Answer from the drawing. Dimensions are ordinates in mm from the lowest x, y and z of the part. Round coordinates to 2 decimals unless told otherwise and drop trailing zeros. Write each loop counter-clockwise with the first axis right and the second up, starting at its lowest first coordinate (ties: lowest second). Pieces come first, ordered by that corner, then holes. Notation, with made-up numbers: (43, 37.5) -> (63, 37.5) arc R13 cw to (63, 51.5) -> close; hole circle Ø4 at (-38, 20.25). An arc over 180 degrees is marked (long way). Return JSON: item names as keys, results as strings. Group by question number.
(1) Straight lines are drawn through the part: line 1 (Y direction, x = 21, z = 4.75); line 2 (Y direction, x = 15.75, z = 1.25); line 3 (Z direction, x = 23.25, y = 8). For each, find the intervals that lie inside material, in ascending order.
(2) A cutting plane is placed at A-A on x = 12.7. Give the vertices of the cut face in (y, z), then the cut area to 3 significant figures.
(3) The mould has two halves that part along X. Classify the marked faces 1, 2, 3 and 4: released by +X, released by -X, zero draft, split by the parting line, or undercut.
(4) Given pin 1 (6 mm diameter, centred on y = 19.5, z = 12.5, fed in from +X), flat-ended and moving along its own axis, determine where the tip first touches the part or whether it passes through.
(5) A cutting plane is placed at C-C on z = 21.75. Give the vertices of the cut face in (x, y).
(6) A cutting plane is placed at D-D on y = 3.5. Give the vertices of the cut face in (x, z), then the cut area to 3 significant figures.
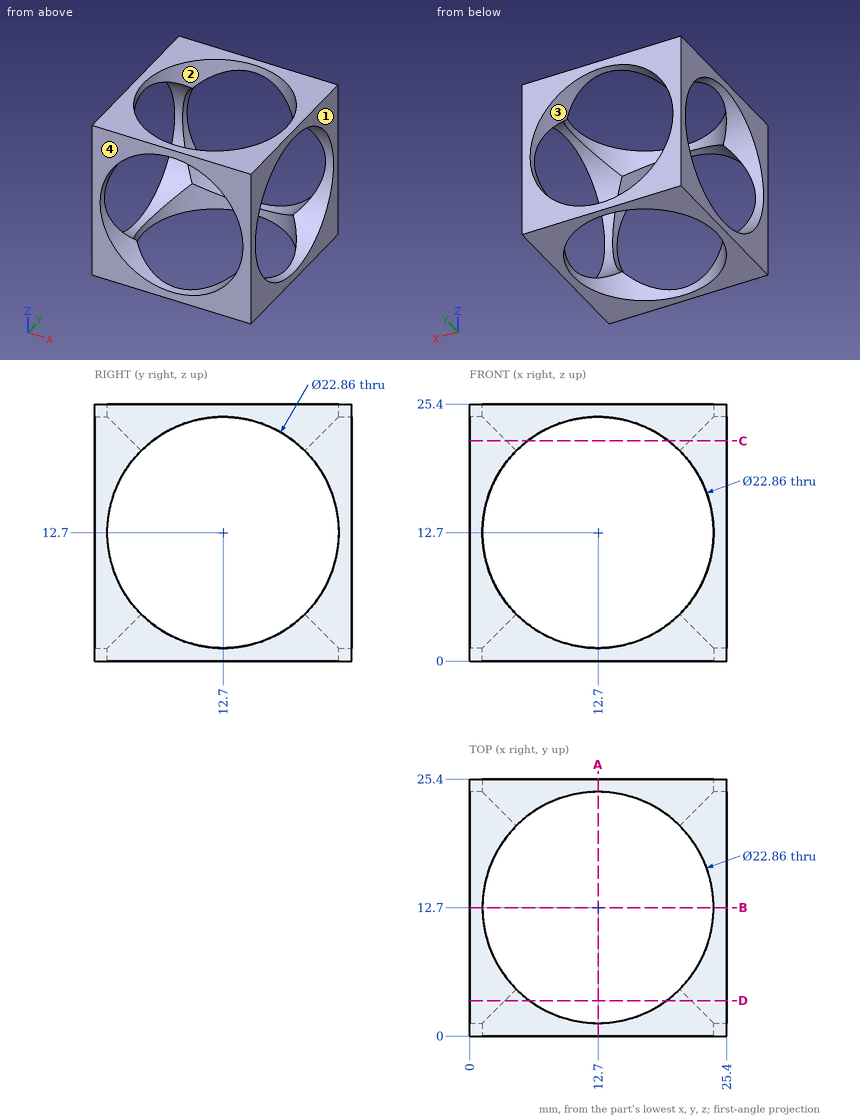
Checks:
{
 "1": {"line 1": "y = 0 to 4.49, 20.91 to 25.4", "line 2": "y = 0 to 1.68, 23.72 to 25.4", "line 3": "z = 0 to 2.28, 23.12 to 25.4"},
 "2": {"outline": "(0, 0) -> (1.27, 0) -> (1.27, 1.27) -> (0, 1.27) -> close; (0, 24.13) -> (1.27, 24.13) -> (1.27, 25.4) -> (0, 25.4) -> close; (24.13, 0) -> (25.4, 0) -> (25.4, 1.27) -> (24.13, 1.27) -> close; (24.13, 24.13) -> (25.4, 24.13) -> (25.4, 25.4) -> (24.13, 25.4) -> close", "area": "6.45 mm^2"},
 "3": {"face 1": "released by +X", "face 2": "undercut", "face 3": "undercut", "face 4": "zero draft"},
 "4": {"pin 1": "passes through"},
 "5": {"outline": "(0, 0) -> (5.72, 0) -> (5.72, 3.65) arc R11.43 cw to (3.65, 5.72) -> (0, 5.72) -> close; (0, 19.68) -> (3.65, 19.68) arc R11.43 cw to (5.72, 21.75) -> (5.72, 25.4) -> (0, 25.4) -> close; (19.68, 0) -> (25.4, 0) -> (25.4, 5.72) -> (21.75, 5.72) arc R11.43 cw to (19.68, 3.65) -> close; (19.68, 21.75) arc R11.43 cw to (21.75, 19.68) -> (25.4, 19.68) -> (25.4, 25.4) -> (19.68, 25.4) -> close"},
 "6": {"outline": "(0, 0) -> (5.92, 0) -> (5.92, 3.5) arc R11.43 cw to (3.5, 5.92) -> (0, 5.92) -> close; (0, 19.48) -> (3.5, 19.48) arc R11.43 cw to (5.92, 21.9) -> (5.92, 25.4) -> (0, 25.4) -> close; (19.48, 0) -> (25.4, 0) -> (25.4, 5.92) -> (21.9, 5.92) arc R11.43 cw to (19.48, 3.5) -> close; (19.48, 21.9) arc R11.43 cw to (21.9, 19.48) -> (25.4, 19.48) -> (25.4, 25.4) -> (19.48, 25.4) -> close", "area": "127 mm^2"}
}
